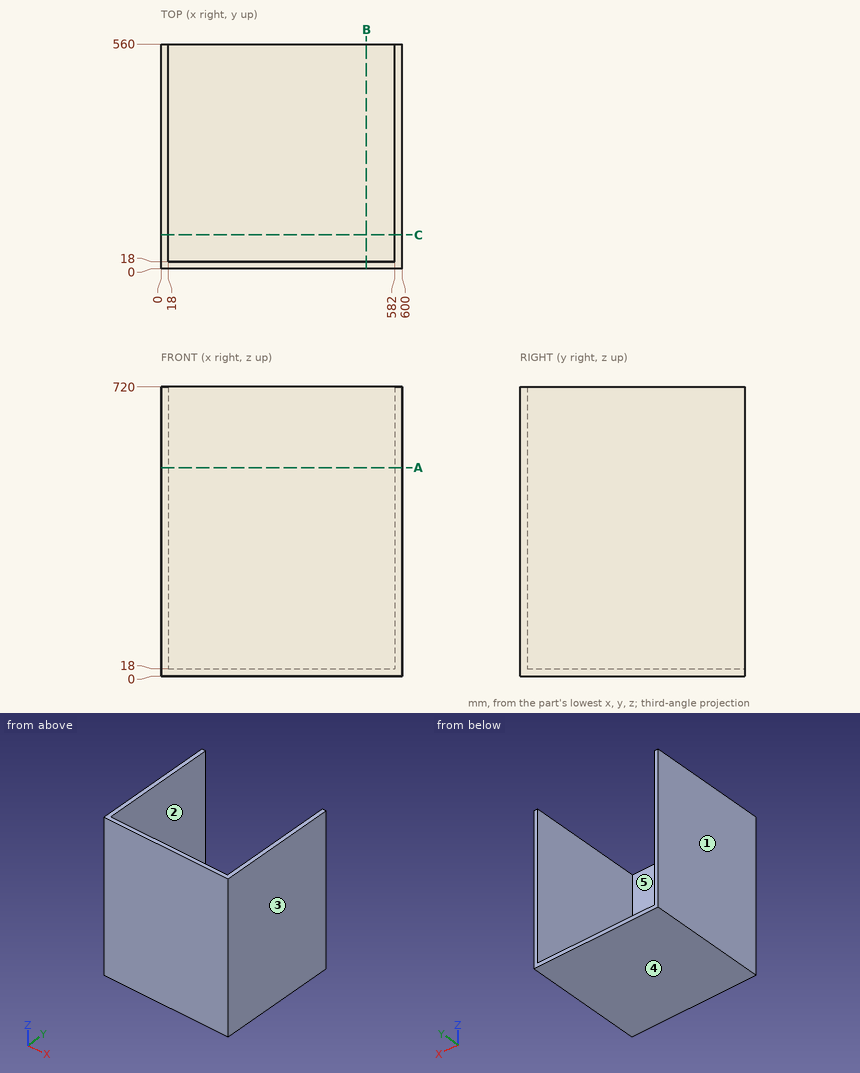
For this review, use the dimensioned drawing (mm, ordinates from the lowest corner) and the shaded views. A direction names the side the tool comes from. Coordinates: 2 decimals unless noted, no trailing zeros. Loops run counter-clockwise (first coordinate to the right, second up) from the corner with the lowest first, then second, coordinate; pieces in that order, holes last. Notation, with made-up numbers: (74, 17.5) -> (112, 17.5) arc R19 ccw to (112, 37.5) -> close; hole circle Ø6 at (-11.75, -7). An arc over 180 degrees is marked (long way). Use a Markdown table: item, result. Add a question column.
1. Machinability: for the marked faces 1 and 2, which of the approach directions +Z, -Z, +X, -X, +Y, -Y give a long, thin tool a straight path to every point of the face, cutting with its end or side? Answer none if there is none.
2. Add section A-A on z = 519. Write out the cut boundary in (x, y), plus the area to 3 significant figures.
3. Add section B-B on x = 511. Write out the cut boundary in (y, z).
4. To check wall thickness, follow line 1 (X direction, y = 189, z = 69); line 2 (Y direction, x = 439.5, z = 108.5). State the ranges of each line that lie inside material, in increasing order.
5. Clearance check with flat-ended pins moving along their axes: pin 1 Ø2 at (x, y) = (109.5, 393.5) entering from +Z; pin 2 Ø1 at (x, z) = (537, 448.5) entering from +Y. State where each tip first meets the part, or that it passes through.
6. Add section C-C on y = 84.5. Write out the cut boundary in (x, z), plus the area to 3 significant figures.
7. Draft analysis for pull direction X (two halves, no side actions). For the marked faces 3, 4 and 5, state which applies: pulls with the +X half, pulls with the -X half, needs draft (parallel to the pull), parting line crosses it, or undercut.
Returned:
| question | item | result |
|---|---|---|
| 1 | face 1 | +Z, -Z, -X, +Y, -Y |
| 1 | face 2 | +Z, +Y |
| 2 | outline | (0, 0) -> (600, 0) -> (600, 560) -> (582, 560) -> (582, 18) -> (18, 18) -> (18, 560) -> (0, 560) -> close |
| 2 | area | 30,300 mm² |
| 3 | outline | (0, 0) -> (560, 0) -> (560, 18) -> (18, 18) -> (18, 720) -> (0, 720) -> close |
| 4 | line 1 | x = 0 to 18, 582 to 600 |
| 4 | line 2 | y = 0 to 18 |
| 5 | pin 1 | stops at z = 18 |
| 5 | pin 2 | stops at y = 18 |
| 6 | outline | (0, 0) -> (600, 0) -> (600, 720) -> (582, 720) -> (582, 18) -> (18, 18) -> (18, 720) -> (0, 720) -> close |
| 6 | area | 36,100 mm² |
| 7 | face 3 | pulls with the +X half |
| 7 | face 4 | needs draft |
| 7 | face 5 | undercut |
